Can you work these out from the model? Positions are in its coordinate system, mm. A direction names the side the tool comes from. Coordinates: 2 decimals unless noted, no trailing zeros. Loops run counter-clockwise (first coordinate to the right, second up) from the corner with the lowest first, then second, coordinate; pieces in that order, holes last.
```python
from build123d import *

# Parameters (mm, degrees)
SKETCH_1_W                       = 343
SKETCH_1_H                       = 18.5
EXTRUDE_1_DEPTH                  = 2
SHEET_METAL_1_OUTLINE_W          = 343
SHEET_METAL_1_OUTLINE_H          = 18.5
SHEET_METAL_1_DEPTH              = 0.5
SM_EDGE_FLANGE_1_STRIP_W         = 8
SM_EDGE_FLANGE_1_STRIP_H         = 1.5
SM_EDGE_FLANGE_1_STRIP_CUT_DEPTH = 343
SM_EDGE_FLANGE_1_DEPTH           = 343
SM_EDGE_FLANGE_2_STRIP_W         = 26.5
SM_EDGE_FLANGE_2_STRIP_H         = 1.5
SM_EDGE_FLANGE_2_STRIP_CUT_DEPTH = 17.5
SM_EDGE_FLANGE_2_DEPTH           = 17.5
SM_EDGE_FLANGE_3_STRIP_W         = 26.5
SM_EDGE_FLANGE_3_STRIP_H         = 1.5
SM_EDGE_FLANGE_3_STRIP_CUT_DEPTH = 17.5
SM_EDGE_FLANGE_3_DEPTH           = 17.5


# Read off the part's stored shape, not the designer's step: Преобразовать-Твердое тело1
# Sheet-metal steps are written as plain solids
with BuildPart() as part:
    # Sketch 1 → Бобышка-Вытянуть1 (new body)
    with BuildSketch(Plane(origin=(0, 0, 0), x_dir=(1, 0, 0), z_dir=(0, 1, 0))):
        with Locations((171.5, 9.25)):
            Rectangle(SKETCH_1_W, SKETCH_1_H)
    extrude(amount=EXTRUDE_1_DEPTH)

    # Sheet Metal 1 outline → Sheet Metal 1 (cut)
    with BuildSketch(Plane(origin=(0, 0, 0), x_dir=(1, 0, 0), z_dir=(0, 1, 0))):
        with Locations((171.5, 9.25)):
            Rectangle(SHEET_METAL_1_OUTLINE_W, SHEET_METAL_1_OUTLINE_H)
    extrude(amount=SHEET_METAL_1_DEPTH, mode=Mode.SUBTRACT)

    # Ребро-кромка1 strip (across the edge) → Ребро-кромка1 strip cut (cut)
    with BuildSketch(Plane(origin=(0, 2, 0), x_dir=(0, 0, -1), z_dir=(1, 0, 0))):
        with Locations((-3, -0.75)):
            Rectangle(SM_EDGE_FLANGE_1_STRIP_W, SM_EDGE_FLANGE_1_STRIP_H)
    extrude(amount=SM_EDGE_FLANGE_1_STRIP_CUT_DEPTH, mode=Mode.SUBTRACT)

    # Ребро-кромка1 section (across the edge) → Ребро-кромка1 (add)
    with BuildSketch(Plane(origin=(0, 2, 0), x_dir=(0, 0, -1), z_dir=(1, 0, 0))):
        with BuildLine():
            Line((-1.5, 1), (-1.5, 18.5))
            Line((-1.5, 18.5), (0, 18.5))
            Line((0, 18.5), (0, 1))
            ThreePointArc((0, 1), (0.292893219, 0.292893219), (1, 0))
            Line((1, 0), (1, -1.5))
            ThreePointArc((1, -1.5), (-0.767766953, -0.767766953), (-1.5, 1))
        make_face()
    extrude(amount=SM_EDGE_FLANGE_1_DEPTH)

    # Ребро-кромка2 strip (across the edge) → Ребро-кромка2 strip cut (cut)
    with BuildSketch(Plane(origin=(18.5, 0.5, -1), x_dir=(1, 0, 0), z_dir=(0, 0, -1))):
        with Locations((-12.25, -0.75)):
            Rectangle(SM_EDGE_FLANGE_2_STRIP_W, SM_EDGE_FLANGE_2_STRIP_H)
    extrude(amount=SM_EDGE_FLANGE_2_STRIP_CUT_DEPTH, mode=Mode.SUBTRACT)

    # Ребро-кромка2 section (across the edge) → Ребро-кромка2 (add)
    with BuildSketch(Plane(origin=(18.5, 0.5, -1), x_dir=(1, 0, 0), z_dir=(0, 0, -1))):
        with BuildLine():
            Line((-1.5, 1), (-1.5, 8.5))
            Line((-1.5, 8.5), (0, 8.5))
            Line((0, 8.5), (0, 1))
            ThreePointArc((0, 1), (0.292893219, 0.292893219), (1, 0))
            Line((1, 0), (1, -1.5))
            ThreePointArc((1, -1.5), (-0.767766953, -0.767766953), (-1.5, 1))
        make_face()
    extrude(amount=SM_EDGE_FLANGE_2_DEPTH)

    # Ребро-кромка3 strip (across the edge) → Ребро-кромка3 strip cut (cut)
    with BuildSketch(Plane(origin=(324.5, 0.5, -18.5), x_dir=(-1, 0, 0), z_dir=(0, 0, 1))):
        with Locations((-12.25, -0.75)):
            Rectangle(SM_EDGE_FLANGE_3_STRIP_W, SM_EDGE_FLANGE_3_STRIP_H)
    extrude(amount=SM_EDGE_FLANGE_3_STRIP_CUT_DEPTH, mode=Mode.SUBTRACT)

    # Ребро-кромка3 section (across the edge) → Ребро-кромка3 (add)
    with BuildSketch(Plane(origin=(324.5, 0.5, -18.5), x_dir=(-1, 0, 0), z_dir=(0, 0, 1))):
        with BuildLine():
            Line((-1.5, 1), (-1.5, 8.5))
            Line((-1.5, 8.5), (0, 8.5))
            Line((0, 8.5), (0, 1))
            ThreePointArc((0, 1), (0.292893219, 0.292893219), (1, 0))
            Line((1, 0), (1, -1.5))
            ThreePointArc((1, -1.5), (-0.767766953, -0.767766953), (-1.5, 1))
        make_face()
    extrude(amount=SM_EDGE_FLANGE_3_DEPTH)


solid = part.part
```
(1) I want a section at A-A on x = 143. Write out the boundary of the cut face in (y, z), then the cut area to 3 significant figures.
Check values:
outline: (0.5, -18.5) - (2, -18.5) - (2, -1) arc R1 cw to (3, 0) - (20.5, 0) - (20.5, 1.5) - (3, 1.5) arc R2.5 ccw to (0.5, -1) - close
area: 56.6 mm2
(2) I want a section at C-C on y = 15.25. Write out the boundary of the cut face in (x, z).
Check values:
outline: (0, 0) - (343, 0) - (343, 1.5) - (0, 1.5) - close
(3) I'm going to push flat-ended pins straight in: pin 1 (2 mm diameter, centred on x = 18, y = -3, fed in from +Z); pin 2 (3 mm diameter, centred on y = 0, z = -9, fed in from +X); pin 3 (1.6 mm diameter, centred on x = 12, y = 1, fed in from -Z). Where does each tip first touch, or does it pass through?
Check values:
pin 1: stops at z = -1
pin 2: stops at x = 326
pin 3: stops at z = -1
(4) If I drill on probe 1 along X at (y, z) = (-6.25, -17.5); probe 2 along Z at (x, y) = (144.5, 9.5); probe 3 along Y at (x, z) = (133, -12), over which ranges is the centre line in solid material (lowest first)?
Check values:
probe 1: x = 17 to 18.5, 324.5 to 326
probe 2: z = 0 to 1.5
probe 3: y = 0.5 to 2
(5) Which directions (+Z, -Z, +X, -X, +Y, -Y) give clear straight access to the entire face, cutting with the end or side of a thin tool? Please do faces 1 (the flat face through (324.5, -4, -10)), 2 (the flat face through (171, 1, -18.5)), 3 (the flat face through (169, 12, 0)).
Check values:
face 1: +Z, -Z, -Y
face 2: -Z, +X, -X, +Y, -Y
face 3: -Z, +X, -X, +Y
(6) I want a section at B-B on z = -15.5. Write out the boundary of the cut face in (x, y), then the cut area to 3 significant figures.
Check values:
outline: (17, -8) - (18.5, -8) - (18.5, -0.5) arc R1 cw to (19.5, 0.5) - (323.5, 0.5) arc R1 cw to (324.5, -0.5) - (324.5, -8) - (326, -8) - (326, -0.5) arc R2.5 ccw to (323.5, 2) - (19.5, 2) arc R2.5 ccw to (17, -0.5) - close
area: 487 mm2
(7) If we mould it in two halves opening along X, with no side actions, what happens to faces 4 (the flat face through (17, -4, -10)), 5 (the flat face through (169, 12, 1.5)), 6 (the flat face through (169, 0.5, -10))? For each: released by +X, released by -X, zero draft, split by the parting line, or undercut.
Check values:
face 4: released by -X
face 5: zero draft
face 6: undercut
